Geometry: final body of the model. Coordinates: model frame, mm. Face numbers are marked on the shaded views. A direction names the side the tool comes from. Give positions to 0.01 mm unless a question says otherwise; leave off trailing zeros. Write each loop counter-clockwise with the first axis right and the second up, starting at its lowest first coordinate (ties: lowest second). Pieces come first, ordered by that corner, then holes. Notation, with made-up numbers: M 39.25,-5 L 95.25,-5 A21 ccw 95.25,11 Z; hole C 66.25,23 d4. An arc over 180 degrees is marked long. Use a Markdown table: item, result. Add a question column.
(1) Reachability of the marked faces 1, 2 and 3 from +Z, -Z, +X, -X, +Y, -Y: full face, straight path, thin tool, end or side. Return the list, or none.
(2) Cut plane C-C (y = -1). State how many separate pieces and enclosed holes the cut face has, plus the area to 3 significant figures.
(3) Pin query (flat end, axial travel): pin 1 Ø1.5 at (x, y) = (35.5, -44.5) entering from +Z; pin 2 Ø1.5 at (x, z) = (29.5, 19.5) entering from +Y; pin 3 Ø21 at (y, z) = (-60.62, 35) entering from -X; pin 4 Ø9.5 at (y, z) = (60.62, 35) entering from +X. Return the tip coordinate at first contact, or that it passes through.
(4) Draft query along Y for the marked faces 4, 5 and 6. Return one class per face: released by +Y, released by -Y, zero draft, split by the parting line, or undercut.
(5) Material intervals for L1, parallel to Z at x = 71.25, y = 0; L2, parallel to Y at x = 36.5, z = -1; L3, parallel to X at y = -38, z = 52, sorted ascending.
(6) Cut plane B-B (x = 39.5). Output: boundary loops of the cut face in (y, z).
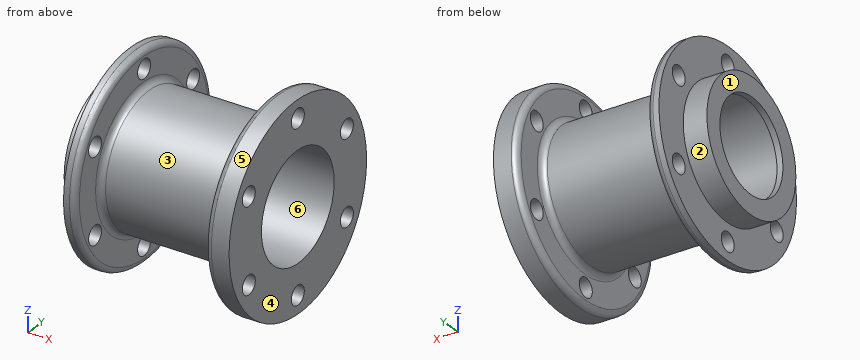
```python
from build123d import *

# Parameters (mm, degrees)
FILLET1_R               = 5
CUT_EXTRUDE1_DEPTH      = 178.059312144
CUT_EXTRUDE1_DEPTH_BACK = 178.059312144
SKETCH2_R               = 8


with BuildPart() as part:
    # Sketch1 → Revolve1 (revolve)
    with BuildSketch(Plane.XY, mode=Mode.PRIVATE) as revolve1_sk:
        Polygon((-80, 55), (-80, 50), (-80, 39), (-75, 39), (-75, 45), (80, 45), (80, 85), (60, 85), (60, 55), (-50, 55), (-50, 85), (-60, 85), (-60, 55), align=None)
    revolve(revolve1_sk.sketch.rotate(Axis((-80, 0, 0), (1, 0, 0)), 180), axis=Axis((-80, 0, 0), (1, 0, 0)))

    # Fillet1
    fillet1_edges = [part.edges().sort_by_distance(p)[0] for p in [
        (-50, 85, 0),
        (-50, 55, 0),
        (60, 55, 0),
        (60, 85, 0),
    ]]
    fillet(fillet1_edges, radius=FILLET1_R)

    # Sketch2 → Cut-Extrude1 (cut, two sides: drawn at the far end of the back side and taken through both)
    with BuildSketch(Plane(origin=(-50, 0, 0), x_dir=(0, 0, -1), z_dir=(1, 0, 0)).offset(-CUT_EXTRUDE1_DEPTH_BACK)):
        with Locations(Location((70, 0, 0), (0, 0, 90))):
            Circle(SKETCH2_R)
        with Locations(Location((35, -60.621778265, 0), (0, 0, 90))):
            Circle(SKETCH2_R)
        with Locations(Location((-35, -60.621778265, 0), (0, 0, 90))):
            Circle(SKETCH2_R)
        with Locations(Location((-70, 0, 0), (0, 0, 90))):
            Circle(SKETCH2_R)
        with Locations(Location((-35, 60.621778265, 0), (0, 0, 90))):
            Circle(SKETCH2_R)
        with Locations(Location((35, 60.621778265, 0), (0, 0, 90))):
            Circle(SKETCH2_R)
    extrude(amount=CUT_EXTRUDE1_DEPTH + CUT_EXTRUDE1_DEPTH_BACK, mode=Mode.SUBTRACT)


solid = part.part
```
Answer list:
| question | item | result |
|---|---|---|
| 1 | face 1 | +Z, -Z, -X, +Y, -Y |
| 1 | face 2 | -X |
| 1 | face 3 | none |
| 2 | separate pieces | 6 |
| 2 | enclosed holes | 0 |
| 2 | area | 4,110 mm² |
| 3 | pin 1 | z = 33.33 |
| 3 | pin 2 | y = 51.71 |
| 3 | pin 3 | x = -60 |
| 3 | pin 4 | through |
| 4 | face 4 | zero draft |
| 4 | face 5 | split by the parting line |
| 4 | face 6 | undercut |
| 5 | L1 | -85 to -78, -62 to -45, 45 to 62, 78 to 85 |
| 5 | L2 | -54.99 to -44.99, 44.99 to 54.99 |
| 5 | L3 | -60 to -50, 60 to 80 |
| 6 | outline | C 0,0 d110; hole C 0,0 d90 |
